Work out the finished part from the listing and answer in its coordinate system (mm). A direction names the side the tool comes from. Coordinates: 2 decimals unless noted, no trailing zeros. Loops run counter-clockwise (first coordinate to the right, second up) from the corner with the lowest first, then second, coordinate; pieces in that order, holes last.
```python
from build123d import *

# Parameters (mm, degrees)
BOSS_EXTRUDE1_DEPTH = 50.8
SKETCH3_R           = 2.38125
CUT_EXTRUDE1_DEPTH  = 15.605


with BuildPart() as part:
    # Sketch1 → Boss-Extrude1 (new body, symmetric)
    with BuildSketch(Plane(origin=(0, 0, 0), x_dir=(0, 0, -1), z_dir=(1, 0, 0))):
        Polygon((0, 11.43), (0, -11.43), (14.605, -11.43), (14.605, -9.652), (1.778, -9.652), (1.778, 9.652), (14.605, 9.652), (14.605, 11.43), align=None)
    extrude(amount=BOSS_EXTRUDE1_DEPTH, both=True)

    # Sketch3 → Cut-Extrude1 (cut, through all)
    with BuildSketch(Plane.XY):
        with Locations((44.45, 0)):
            Circle(SKETCH3_R)
    cut_extrude1 = extrude(amount=-CUT_EXTRUDE1_DEPTH, mode=Mode.SUBTRACT)

    # Mirror1: Cut-Extrude1 across plane
    add(cut_extrude1.mirror(Plane(origin=(0, 0, 0), x_dir=(0, 0, 1), z_dir=(1, 0, 0))), mode=Mode.SUBTRACT)


solid = part.part
```
1. A cutting plane is placed at D-D, the plane x = 28. Give the vertices of the cut face in (y, z) (3 decimals).
2. For faces 5 (the flat face through (1, -9.652, -8)), 6 (the flat face through (1, 11, -14.605)), determine the directions among +Z, -Z, +X, -X, +Y, -Y from which every point of the face is accessible in a straight line to the end or side of a thin tool.
3. A cutting plane is placed at A-A, the plane y = 0. Give the vertices of the cut face in (x, z).
4. Straight lines are drawn through the part: probe 1 along Y at (x, z) = (9.5, -12.5); probe 2 along Z at (x, y) = (6, -6.75). For each, find the intervals that lie inside material, in ascending order.
5. This flat-tipped pin is pushed along its axis until it touches: P1, Ø6, axis at x = -21.5, y = -4, coming from the -Z side. Where does it stop, or does it pass through?
6. A cutting plane is placed at B-B, the plane z = -10. Give the vertices of the cut face in (x, y), then the cut area to 3 significant figures.
7. Determine the mould class of faces 1 (the flat face through (1, 0, -1.778)), 2 (the cylindrical face through (-46.65, -0.91, -0.88)), 3 (the flat face through (1, 11.43, -7)), 4 (the flat face through (-50.8, 0, -1)) for opening direction Y: released by +Y, released by -Y, zero draft, split by the parting line, or undercut.
8. A cutting plane is placed at C-C, the plane x = 44.45. Give the vertices of the cut face in (y, z) (3 decimals), then the cut area to 3 significant figures.
Answers below:
1. outline: (-11.43, -14.605) - (-9.652, -14.605) - (-9.652, -1.778) - (9.652, -1.778) - (9.652, -14.605) - (11.43, -14.605) - (11.43, 0) - (-11.43, 0) - close
2. face 5: -Z, +X, -X
2. face 6: -Z, +X, -X, +Y, -Y
3. outline: (-50.8, -1.78) - (-46.83, -1.78) - (-46.83, 0) - (-50.8, 0) - close; (-42.07, -1.78) - (42.07, -1.78) - (42.07, 0) - (-42.07, 0) - close; (46.83, -1.78) - (50.8, -1.78) - (50.8, 0) - (46.83, 0) - close
4. probe 1: y = -11.43 to -9.65, 9.65 to 11.43
4. probe 2: z = -1.78 to 0
5. P1: stops at z = -1.78
6. outline: (-50.8, -11.43) - (50.8, -11.43) - (50.8, -9.65) - (-50.8, -9.65) - close; (-50.8, 9.65) - (50.8, 9.65) - (50.8, 11.43) - (-50.8, 11.43) - close
6. area: 361 mm2
7. face 1: undercut
7. face 2: undercut
7. face 3: released by +Y
7. face 4: zero draft
8. outline: (-11.43, -14.605) - (-9.652, -14.605) - (-9.652, -1.778) - (-2.381, -1.778) - (-2.381, 0) - (-11.43, 0) - close; (2.381, -1.778) - (9.652, -1.778) - (9.652, -14.605) - (11.43, -14.605) - (11.43, 0) - (2.381, 0) - close
8. area: 77.8 mm2
